Verification items for the finished model (mm, model axes). A direction names the side the tool comes from. Round coordinates to 2 decimals unless told otherwise and drop trailing zeros. Order: outer loops, then holes, each group sorted by start corner. A loop starts at its lowest first (then second) coordinate and runs counter-clockwise, first axis right, second up.
```python
from build123d import *

# Parameters (mm, degrees)
SKETCH1_R           = 24.25
SKETCH1_R_2         = 14.25
BOSS_EXTRUDE1_DEPTH = 25
SKETCH2_R           = 24.25
SKETCH2_R_2         = 1.8
BOSS_EXTRUDE2_DEPTH = 4
SKETCH3_W           = 5
SKETCH3_H           = 8.89
CUT_EXTRUDE1_DEPTH  = 11
SKETCH4_R           = 1.27
CUT_EXTRUDE2_DEPTH  = 39
FILLET1_R           = 4
SKETCH5_R           = 1.27
CUT_EXTRUDE3_DEPTH  = 78


with BuildPart() as part:
    # Sketch1 → Boss-Extrude1 (new body)
    with BuildSketch(Plane.XY):
        Circle(SKETCH1_R)
        Circle(SKETCH1_R_2, mode=Mode.SUBTRACT)
    extrude(amount=BOSS_EXTRUDE1_DEPTH)

    # Sketch2 → Boss-Extrude2 (add)
    with BuildSketch(Plane.XY.offset(25)):
        Circle(SKETCH2_R)
        Circle(SKETCH2_R_2, mode=Mode.SUBTRACT)
    extrude(amount=BOSS_EXTRUDE2_DEPTH)

    # Sketch3 → Cut-Extrude1 (cut)
    with BuildSketch(Plane(origin=(0, 0, 0), x_dir=(-1, 0, 0), z_dir=(0, 0, -1))):
        with Locations((-18.5, 0)):
            Rectangle(SKETCH3_W, SKETCH3_H)
        with Locations((18.5, 0)):
            Rectangle(SKETCH3_W, SKETCH3_H)
    extrude(amount=-CUT_EXTRUDE1_DEPTH, mode=Mode.SUBTRACT)

    # Sketch4 → Cut-Extrude2 (cut, symmetric)
    with BuildSketch(Plane(origin=(0, 0, 0), x_dir=(0, 0, -1), z_dir=(1, 0, 0))):
        with Locations((-4.5, 0)):
            Circle(SKETCH4_R)
    extrude(amount=CUT_EXTRUDE2_DEPTH, both=True, mode=Mode.SUBTRACT)

    # Fillet1
    fillet1_edges = [part.edges().sort_by_distance(p)[0] for p in [
        (-14.25, 0, 25),
    ]]
    fillet(fillet1_edges, radius=FILLET1_R)

    # Sketch5 → Cut-Extrude3 (cut)
    with BuildSketch(Plane.XY.offset(29)):
        with Locations((0, 10)):
            Circle(SKETCH5_R)
        with Locations((7.071067812, 7.071067812)):
            Circle(SKETCH5_R)
        with Locations((10, 0)):
            Circle(SKETCH5_R)
        with Locations((7.071067812, -7.071067812)):
            Circle(SKETCH5_R)
        with Locations((0, -10)):
            Circle(SKETCH5_R)
        with Locations((-7.071067812, -7.071067812)):
            Circle(SKETCH5_R)
        with Locations((-10, 0)):
            Circle(SKETCH5_R)
        with Locations((-7.071067812, 7.071067812)):
            Circle(SKETCH5_R)
    extrude(amount=-CUT_EXTRUDE3_DEPTH, mode=Mode.SUBTRACT)


solid = part.part
```
1) Sectioned sample at A-A on x = 0. Record the cut outline in (y, z), then the cut area to 3 significant figures.
2) Tool access check on faces 1 (the cylindrical face through (22.4, -9.29, 14.3)), 2 (the cylindrical face through (13.163, -5.458, 10.353)). Record the directions out of +Z, -Z, +X, -X, +Y, -Y that give a thin tool (end or side, any length) a straight path to the whole face; none if there is none.
3) Draft check along Z on faces 3 (the flat face through (-18, 0, 11)), 4 (the cylindrical face through (-15.08, 0.38, 3.29)), 5 (the cylindrical face through (11.17, -0.49, 26.96)). Enter one of: released by +Z, released by -Z, zero draft, split by the parting line, or undercut.
4) Sectioned sample at C-C on y = 0. Count the separate pieces of the cut face and the enclosed holes in it, then the cut area to 3 significant figures.
5) Sectioned sample at D-D on x = -18.5. Record the cut outline in (y, z) (3 decimals), then the cut area to 3 significant figures.
6) Go/stop test with flat-tipped pins: pin 1 Ø1 at (x, z) = (7, 8) entering from -Y; pin 2 Ø10 at (y, z) = (11, 17) entering from -X; pin 3 Ø2 at (y, z) = (-4.5, 25.5) entering from -X; pin 4 Ø2 at (x, y) = (-7.07, -7.07) entering from +Z. Record where each tip stops, or that it passes through.
7) Scan lines: probe 1 along Y at (x, z) = (0, 15.75); probe 2 along X at (y, z) = (2.5, 6.5); probe 3 along Y at (x, z) = (7, 27). Record each from-to range of solid material in increasing order.
Returned:
1. outline: (-24.25, 0) - (-14.25, 0) - (-14.25, 21) arc R4 cw to (-11.27, 24.87) - (-11.27, 29) - (-24.25, 29) - close; (-8.73, 25) - (-1.8, 25) - (-1.8, 29) - (-8.73, 29) - close; (1.8, 25) - (8.73, 25) - (8.73, 29) - (1.8, 29) - close; (11.27, 24.87) arc R4 cw to (14.25, 21) - (14.25, 0) - (24.25, 0) - (24.25, 29) - (11.27, 29) - close
1. area: 666 mm2
2. face 1: +Z, -Z
2. face 2: -Z
3. face 3: released by -Z
3. face 4: undercut
3. face 5: zero draft
4. separate pieces: 8
4. enclosed holes: 0
4. area: 531 mm2
5. outline: (-15.678, 0) - (-4.445, 0) - (-4.445, 11) - (4.445, 11) - (4.445, 0) - (15.678, 0) - (15.678, 29) - (-15.678, 29) - close
5. area: 812 mm2
6. pin 1: stops at y = -23.36
6. pin 2: stops at x = -23.5
6. pin 3: stops at x = -24
6. pin 4: passes through
7. probe 1: y = -24.25 to -14.25, 14.25 to 24.25
7. probe 2: x = -24.12 to -21, -16 to -14.03, 14.03 to 16, 21 to 24.12
7. probe 3: y = -23.22 to -8.34, -5.8 to 5.8, 8.34 to 23.22
